```python
from build123d import *

# Parameters (mm, degrees)
F0_R      = 10
F1_DEPTH  = 30.5
F2_R      = 6
F3_DEPTH  = 20
F4_R      = 6
F5_DEPTH  = 34
F7_W      = 4
F7_H      = 23
F8_DEPTH  = 2.5
F9_R      = 1.9999
F10_W     = 4
F10_H     = 20
F11_DEPTH = 25
F12_R     = 1.9999
F13_SIZE  = 0.5


# Not quite as in the source:
# - a fillet or chamfer is up to 0.001 mm smaller than in the source, because OpenCascade refuses the exact size


with BuildPart() as f1:
    # F0 (on Front) → F1 (new body)
    with BuildSketch(Plane.XZ):
        Circle(F0_R)
    extrude(amount=F1_DEPTH)

    # F2 (on face) → F3 (cut)
    with BuildSketch(Plane.XZ.offset(30.5)):
        Circle(F2_R)
    extrude(amount=-F3_DEPTH, mode=Mode.SUBTRACT)

    # F4 (on face) → F5 (join)
    with BuildSketch(Plane(origin=(0, 0, 0), x_dir=(-1, 0, 0), z_dir=(0, 1, 0))):
        Circle(F4_R)
    extrude(amount=F5_DEPTH)

    # F7 (on offset) → F8 (cut)
    with BuildSketch(Plane.XY.offset(-6)):
        with Locations((0, 22.5)):
            Rectangle(F7_W, F7_H)
    extrude(amount=F8_DEPTH, mode=Mode.SUBTRACT)

    # F9 (radius 2 in the source; OpenCascade refuses exactly that, so slightly less here)
    f9_edges = [f1.edges().sort_by_distance(p)[0] for p in [
        (-2, 11, -4.578427),
        (2, 11, -4.578427),
    ]]
    fillet(f9_edges, radius=F9_R)

    # F10 (on Top) → F11 (cut)
    with BuildSketch(Plane.XY):
        with Locations((0, -20.5)):
            Rectangle(F10_W, F10_H)
    extrude(amount=-F11_DEPTH, mode=Mode.SUBTRACT)

    # F12 (radius 2 in the source; OpenCascade refuses exactly that, so slightly less here)
    f12_edges = [f1.edges().sort_by_distance(p)[0] for p in [
        (2, -10.5, -7.727407),
        (-2, -10.5, -7.727407),
    ]]
    fillet(f12_edges, radius=F12_R)

    # F13
    f13_edges = [f1.edges().sort_by_distance(p)[0] for p in [
        (-10, 0, 0),
        (3.464102, 34, 4.898979),
        (-6.324555, -30.5, 7.745967),
    ]]
    chamfer(f13_edges, length=F13_SIZE)


solid = f1.part
```
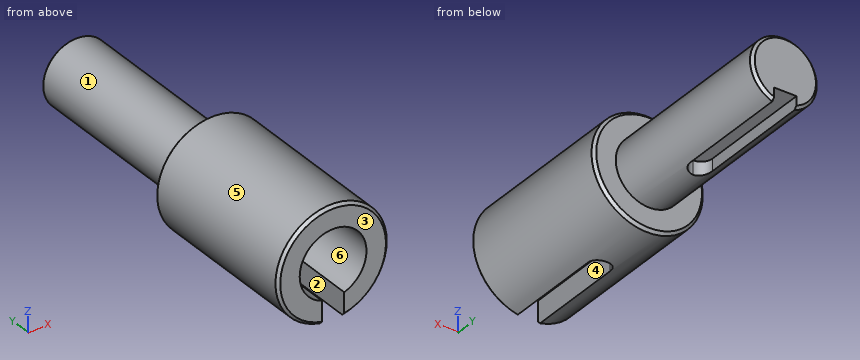
Read the model definition and answer for the solid it produces. Units are mm, in the model's axes. Face numbers are marked on the shaded views. A direction names the side the tool comes from. Give positions to 0.01 mm unless a question says otherwise; leave off trailing zeros. Order: outer loops, then holes, each group sorted by start corner. A loop starts at its lowest first (then second) coordinate and runs counter-clockwise, first axis right, second up.
(1) Find section D-D (y = 25.5). Give the vertices of the cut face in (x, z), plus the area to 3 significant figures.
(2) For the marked faces 1, 2 and 3, determine the directions among +Z, -Z, +X, -X, +Y, -Y from which every point of the face is accessible in a straight line to the end or side of a thin tool.
(3) Find section A-A (z = 0). Give the vertices of the cut face in (x, y), plus the area to 3 significant figures.
(4) For a pull along Z with two mould halves and no side action, classify the marked faces 4, 5 and 6 as released by +Z, released by -Z, zero draft, split by the parting line, or undercut.
(5) Straight lines are drawn through the part: L1, parallel to X at y = -25.5, z = 0; L2, parallel to Y at x = 6.25, z = 4.5; L3, parallel to Y at x = -1, z = -2.5. For each, find the intervals that lie inside material, in ascending order.
(6) Given pin 1 (2.5 mm diameter, centred on y = 26, z = -4.5, fed in from -X); pin 2 (4 mm diameter, centred on y = 21, z = 4.5, fed in from +X); pin 3 (9.5 mm diameter, centred on x = -0.5, z = -4.5, fed in from -Y); pin 4 (2 mm diameter, centred on x = 0.5, y = 28, fed in from -Z), each flat-ended and moving along its own axis, determine where each tip first touches the part or whether it passes through.
(7) Find section C-C (y = -2). Give the vertices of the cut face in (x, z).
(8) Find section B-B (y = -19). Give the vertices of the cut face in (x, z).
Result sheet:
1. outline: (-2, -5.66) - (-2, -3.5) - (2, -3.5) - (2, -5.66) arc R6 ccw (long way) to start
1. area: 104 mm2
2. face 1: +Y
2. face 2: -Z, -Y
2. face 3: +Z, -Z, +X, -X, -Y
3. outline: (-10, -30) - (-9.5, -30.5) - (-6, -30.5) - (-6, -10.5) - (6, -10.5) - (6, -30.5) - (9.5, -30.5) - (10, -30) - (10, -0.5) - (9.5, 0) - (6, 0) - (6, 33.5) - (5.5, 34) - (-5.5, 34) - (-6, 33.5) - (-6, 0) - (-9.5, 0) - (-10, -0.5) - close
3. area: 777 mm2
4. face 4: zero draft
4. face 5: split by the parting line
4. face 6: undercut
5. L1: x = -10 to -6, 6 to 10
5. L2: y = -30.5 to 0
5. L3: y = -10.5 to 34
6. pin 1: stops at x = -5.04
6. pin 2: stops at x = 5.45
6. pin 3: stops at y = -30.5
6. pin 4: stops at z = -3.5
7. outline: circle Ø20 at (0, 0)
8. outline: (-2, -9.8) - (-2, -5.66) arc R6 cw (long way) to (2, -5.66) - (2, -9.8) arc R10 ccw (long way) to start
